from build123d import *

# Parameters (mm, degrees)
SKETCH_1_W                  = 65
SKETCH_1_H                  = 100
EXTRUDE_1_DEPTH             = 5
SKETCH_2_R                  = 1.6
CUT_EXTRUDE_1_DEPTH         = 5
PATTERN_LINEAR_1_COUNT      = 2
PATTERN_LINEAR_1_PITCH      = 75
PATTERN_LINEAR_1_COUNT_DIR2 = 2
PATTERN_LINEAR_1_PITCH_DIR2 = 110
FILLET_1_R                  = 5
SKETCH_4_R                  = 1.65
CUT_EXTRUDE_2_DEPTH         = 31


with BuildPart() as part:
    # Эскиз1 → Бобышка-Вытянуть1 (new body)
    with BuildSketch(Plane.XY):
        Polygon((-35, -48), (-35, -58), (50, -73), (130, -73), (215, -58), (215, -48), (215, 62), (215, 72), (115, 191.360256276), (65, 191.360256276), (-35, 72), (-35, 62), align=None)
        with Locations((90, 62)):
            Rectangle(SKETCH_1_W, SKETCH_1_H, mode=Mode.SUBTRACT)
    extrude(amount=EXTRUDE_1_DEPTH)

    # Эскиз2 → Вырез-Вытянуть1 (cut)
    with BuildSketch(Plane.XY.offset(5)):
        with Locations((52.5, 7)):
            Circle(SKETCH_2_R)
    cut_extrude_1 = extrude(amount=-CUT_EXTRUDE_1_DEPTH, mode=Mode.SUBTRACT)

    # Линейный массив1: Cut-Extrude 1 2 × 2
    with Locations(*[(i * PATTERN_LINEAR_1_PITCH, j * PATTERN_LINEAR_1_PITCH_DIR2, 0) for i in range(PATTERN_LINEAR_1_COUNT) for j in range(PATTERN_LINEAR_1_COUNT_DIR2) if (i, j) != (0, 0)]):
        add(cut_extrude_1, mode=Mode.SUBTRACT)

    # Скругление1
    fillet_1_edges = [part.edges().sort_by_distance(p)[0] for p in [
        (122.5, 112, 2.5),
        (57.5, 112, 2.5),
        (57.5, 12, 2.5),
        (122.5, 12, 2.5),
    ]]
    fillet(fillet_1_edges, radius=FILLET_1_R)

    # Эскиз4 → Вырез-Вытянуть2 (cut)
    with BuildSketch(Plane(origin=(0, 0, 0), x_dir=(-1, 0, 0), z_dir=(0, 0, -1))):
        with Locations((-16.471095772, -33)):
            Circle(SKETCH_4_R)
        with Locations((-28.528904228, -10.64)):
            Circle(SKETCH_4_R)
        with Locations((-28.75, 22.36)):
            Circle(SKETCH_4_R)
        with Locations((-28.75, 10.36)):
            Circle(SKETCH_4_R)
        with Locations((-45.245579603, 91.884303707)):
            Circle(SKETCH_4_R)
        with Locations((-50.274277733, 102.779816321)):
            Circle(SKETCH_4_R)
        with Locations((-131.821084869, 98.239864017)):
            Circle(SKETCH_4_R)
        with Locations((-136.849782999, 87.344351403)):
            Circle(SKETCH_4_R)
        with Locations((-151.471095772, -10.64)):
            Circle(SKETCH_4_R)
        with Locations((-163.528904228, -33)):
            Circle(SKETCH_4_R)
        with Locations((-151.25, 22.36)):
            Circle(SKETCH_4_R)
        with Locations((-151.25, 10.36)):
            Circle(SKETCH_4_R)
    extrude(amount=-CUT_EXTRUDE_2_DEPTH, mode=Mode.SUBTRACT)


solid = part.part
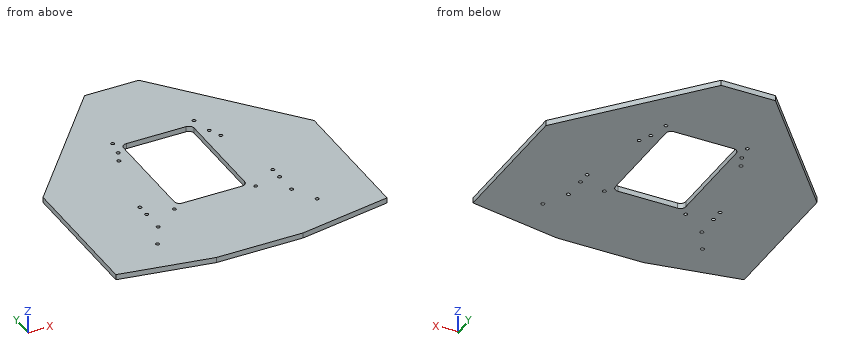
Can you work these out from the model? Positions are in its coordinate system, mm. Give positions to 0.01 mm unless a question says otherwise; leave off trailing zeros. Loops run counter-clockwise (first coordinate to the right, second up) from the corner with the lowest first, then second, coordinate; pieces in that order, holes last. Notation, with made-up numbers: (54, 11) -> (106, 11) arc R28 cw to (106, 50) -> close; hole circle Ø11 at (51, 31). An arc over 180 degrees is marked (long way). Use one line per item in the form item = value.
1) Will these pins go through, and if not, where does the flat tip stop? pin 1 (4.5 mm diameter, centred on x = 151.25, y = 10.36, fed in from +Z); pin 2 (3 mm diameter, centred on x = 151.25, y = 22.36, fed in from +Z).
Answers:
pin_1 = 5
pin_2 = through
2) If we section it at D-D (x = 22): Please give me the cut outline in (y, z).
Answers:
outline = (-68.06, 0) -> (140.04, 0) -> (140.04, 5) -> (-68.06, 5) -> close
3) If we section it at B-B (z = 3.35): Count the separate pieces of the cut face and the enclosed holes in it, plus the area to 3 significant figures.
Answers:
separate_pieces = 1
enclosed_holes = 17
area = 46,300 mm²
4) If we section it at C-C (x = 180): Please give me the cut outline in (y, z).
Answers:
outline = (-64.18, 0) -> (113.78, 0) -> (113.78, 5) -> (-64.18, 5) -> close
5) If we section it at A-A (x = 112): Please give me the cut outline in (y, z), plus the area to 3 significant figures.
Answers:
outline = (-73, 0) -> (12, 0) -> (12, 5) -> (-73, 5) -> close; (112, 0) -> (191.36, 0) -> (191.36, 5) -> (112, 5) -> close
area = 822 mm²
6) I need wall thicknesses on line 1 along Y through (x, z) = (127.5, 2.9); line 2 along X through (y, z) = (48.5, 4); line 3 along Y through (x, z) = (76, 2.8). Which ranges of each line are inside material? Lowest first, please.
Answers:
line_1 = -73 to 5.4, 8.6 to 115.4, 118.6 to 176.44
line_2 = -35 to 57.5, 122.5 to 215
line_3 = -73 to 12, 112 to 191.36
